```python
from build123d import *

# Parameters (mm, degrees)
F0_W      = 63.5
F0_H      = 63.5
F1_DEPTH  = 171.45
F3_W      = 31.75
F3_H      = 31.75
F1_FACE_W = 63.5
F1_FACE_H = 63.5
F6_DEPTH  = 19.05
F8_DEPTH  = 19.05


with BuildPart() as f1:
    # F0 (on Top) → F1 (new body)
    with BuildSketch(Plane.XY):
        Rectangle(F0_W, F0_H)
    extrude(amount=-F1_DEPTH)

    # F3 (on offset) → F4 section 0
    with BuildSketch(Plane(origin=(0, 0, -374.65), x_dir=(1, 0, 0), z_dir=(0, 0, -1))):
        with Locations((-15.875, -15.875)):
            Rectangle(F3_W, F3_H)
    # F1_face (on face) → F4 section 1
    with BuildSketch(Plane(origin=(0, 0, -171.45), x_dir=(1, 0, 0), z_dir=(0, 0, -1))):
        Rectangle(F1_FACE_W, F1_FACE_H)
    loft()

    # F5 (on face) → F6 (cut)
    with BuildSketch(Plane.XZ.offset(31.75)):
        with BuildLine():
            Line((-22.225, -19.05), (-22.225, -31.75))
            ThreePointArc((-22.225, -31.75), (-15.875, -38.1), (-9.525, -31.75))
            Line((-9.525, -31.75), (-9.525, -19.05))
            ThreePointArc((-9.525, -19.05), (-15.875, -12.7), (-22.225, -19.05))
        make_face()
    extrude(amount=-F6_DEPTH, mode=Mode.SUBTRACT)

    # F7 (on face) → F8 (cut)
    with BuildSketch(Plane.YZ.offset(31.75)):
        with BuildLine():
            Line((9.525, -19.05), (9.525, -31.75))
            ThreePointArc((9.525, -31.75), (15.875, -38.1), (22.225, -31.75))
            Line((22.225, -31.75), (22.225, -19.05))
            ThreePointArc((22.225, -19.05), (15.875, -12.7), (9.525, -19.05))
        make_face()
    extrude(amount=-F8_DEPTH, mode=Mode.SUBTRACT)


solid = f1.part
```
Part model, mm, in its own coordinate system. A direction names the side the tool comes from. Round coordinates to 2 decimals unless told otherwise and drop trailing zeros. Return JSON: item names as keys, results as strings. Group by question number.
Q1. Probe L1, parallel to Y at x = 28.5, z = -25.5 (3 decimals); L2, parallel to X at y = -3, z = -209; L3, parallel to Y at x = -5, z = -306. List the from-to ranges inside material, lowest first. Write a range as [from, to].
Q2. Mould opens along X. For faces 1 (the flat face through (-31.75, 8, -184)), 2 (the cylindrical face through (-16, -22.4, -38.1)), 3 (the flat face through (12.7, 16, -25)) say: pulls with the +X half, pulls with the -X half, needs draft (parallel to the pull), parting line crosses it, or undercut.
Q3. Pin check, flat tips, straight feed: pin 1 (4 mm diameter, centred on y = 12.5, z = -26.5, fed in from +X); pin 2 (12 mm diameter, centred on y = 9, z = -284.5, fed in from +X); pin 3 (14 mm diameter, centred on x = -16.5, z = -24.5, fed in from -Y); pin 4 (12 mm diameter, centred on x = -18, z = -286, fed in from -Y). Stop position of each tip, or through.
Q4. Which spindle directions (+Z, -Z, +X, -X, +Y, -Y) get a long thin tool onto all of the face, cutting with end or side? Do faces 4 (the flat face through (22, 9.525, -25)), 5 (the flat face through (31.75, 0, -85)), 6 (the cylindrical face through (-15.74, -22.36, -12.7)). Say none if no direction does.
Answer:
{
 "1": {"L1": "[-31.75, 9.525], [22.225, 31.75]", "L2": "[-31.75, 25.88]", "L3": "[-10.73, 31.75]"},
 "2": {"face 1": "pulls with the -X half", "face 2": "undercut", "face 3": "pulls with the +X half"},
 "3": {"pin 1": "x = 12.7", "pin 2": "x = 15.02", "pin 3": "y = -31.75", "pin 4": "y = -14.79"},
 "4": {"face 4": "+X", "face 5": "+Z, -Z, +X, +Y, -Y", "face 6": "-Y"}
}
